Model file for the job. Use its own axes, mm. A direction names the side the tool comes from. Round coordinates to 2 decimals unless told otherwise and drop trailing zeros. Loops run counter-clockwise (first coordinate to the right, second up) from the corner with the lowest first, then second, coordinate; pieces in that order, holes last. Notation, with made-up numbers: M 7.5,-7 L 31.5,-7 A9 ccw 31.5,8 Z; hole C -20.75,49 d8. An arc over 180 degrees is marked long. Answer in a Markdown table with one row per item.
from build123d import *
from OCP.BRepFilletAPI import BRepFilletAPI_MakeChamfer

# Parameters (mm, degrees)
SKETCH_1_W             = 23
SKETCH_1_H             = 37.8
EXTRUDE_1_DEPTH        = 16.4
SKETCH_19_W            = 29
SKETCH_19_H            = 16
EXTRUDE_3_DEPTH        = 6
SKETCH_5_W             = 4
SKETCH_5_H             = 5
EXTRUDE_2_DEPTH        = 13.2
SKETCH_20_W            = 2.9
SKETCH_20_H            = 1.2
SKETCH_20_W_2          = 5.1
EXTRUDE_4_DEPTH        = 5
HOLE_WIZARD_M2_5_1_D   = 2.05
HOLE_WIZARD_M3_6_D     = 2.5
HOLE_WIZARD_M3_6_DEPTH = 7.5
HOLE_WIZARD_M3_6_TIP   = 0.751075774
HOLE_WIZARD_M3_7_D     = 2.5
HOLE_WIZARD_M3_7_DEPTH = 7.5
HOLE_WIZARD_M3_7_TIP   = 0.751075774
HOLE_WIZARD_M3_5_D     = 2.5
SKETCH_15_R            = 5.5
CUT_EXTRUDE_4_DEPTH    = 1.5
HOLE_WIZARD_M3_4_D     = 2.5
HOLE_WIZARD_M3_4_DEPTH = 7.5
HOLE_WIZARD_M3_4_TIP   = 0.751075774
CUT_EXTRUDE_5_REACH    = 66.761
CHAMFER_1_SIZE         = 0.5
CHAMFER_1_SIZE2        = 0.288675135
CHAMFER_2_SIZE         = 0.5
CHAMFER_2_SIZE2        = 0.288675135
SKETCH_25_W            = 10
SKETCH_25_H            = 0.4
CUT_EXTRUDE_6_DEPTH    = 37.8
CHAMFER_3_SIZE         = 0.5


with BuildPart() as part:
    # 草图1 → 拉伸1 (new body)
    with BuildSketch(Plane.XY):
        with Locations((11.5, 18.9)):
            Rectangle(SKETCH_1_W, SKETCH_1_H)
    extrude(amount=EXTRUDE_1_DEPTH)

    # 草图19 → 拉伸3 (add)
    with BuildSketch(Plane.XZ):
        with Locations((11.5, 8.2)):
            Rectangle(SKETCH_19_W, SKETCH_19_H)
    extrude(amount=EXTRUDE_3_DEPTH)

    # 草图5 → 拉伸2 (add)
    with BuildSketch(Plane.XZ.offset(6)):
        with Locations((3.9, 8.2)):
            Rectangle(SKETCH_5_W, SKETCH_5_H)
        with Locations((19.1, 8.2)):
            Rectangle(SKETCH_5_W, SKETCH_5_H)
    extrude(amount=EXTRUDE_2_DEPTH)

    # 草图20 → 拉伸4 (add)
    with BuildSketch(Plane.XY.offset(10.7)):
        with Locations((0.45, -6.6)):
            Rectangle(SKETCH_20_W, SKETCH_20_H)
        with Locations((8.45, -6.6)):
            Rectangle(SKETCH_20_W_2, SKETCH_20_H)
        with Locations((14.55, -6.6)):
            Rectangle(SKETCH_20_W_2, SKETCH_20_H)
        with Locations((22.55, -6.6)):
            Rectangle(SKETCH_20_W, SKETCH_20_H)
    extrude(amount=-EXTRUDE_4_DEPTH)

    # M2.5 螺纹孔1 (through all)
    with Locations(Plane(origin=(21.1, 0, 0), x_dir=(0, 0, -1), z_dir=(1, 0, 0))):
        with Locations((-8.2, -16.2), (-8.2, -10.5)):
            Hole(HOLE_WIZARD_M2_5_1_D / 2)

    # M3 螺纹孔6
    with Locations(Plane(origin=(23, 0, 0), x_dir=(0, 0, -1), z_dir=(1, 0, 0))):
        with Locations((-2.7, 28.8), (-13.7, 18.8)):
            Hole(HOLE_WIZARD_M3_6_D / 2, depth=HOLE_WIZARD_M3_6_DEPTH)
            with Locations((0, 0, -(HOLE_WIZARD_M3_6_DEPTH + HOLE_WIZARD_M3_6_TIP / 2))):  # 118° drill point
                Cone(0, HOLE_WIZARD_M3_6_D / 2, HOLE_WIZARD_M3_6_TIP, mode=Mode.SUBTRACT)

    # M3 螺纹孔7
    with Locations(Plane.ZY):
        with Locations((2.5, 10.8), (13.9, 10.8)):
            Hole(HOLE_WIZARD_M3_7_D / 2, depth=HOLE_WIZARD_M3_7_DEPTH)
            with Locations((0, 0, -(HOLE_WIZARD_M3_7_DEPTH + HOLE_WIZARD_M3_7_TIP / 2))):  # 118° drill point
                Cone(0, HOLE_WIZARD_M3_7_D / 2, HOLE_WIZARD_M3_7_TIP, mode=Mode.SUBTRACT)

    # M3 螺纹孔5 (through all)
    with Locations(Plane.XY.offset(16.4)):
        with Locations((3.5, 14.8), (19.5, 14.8)):
            Hole(HOLE_WIZARD_M3_5_D / 2)

    # 草图15 → 切除-拉伸4 (cut)
    with BuildSketch(Plane(origin=(0, 37.8, 0), x_dir=(1, 0, 0), z_dir=(0, 1, 0))):
        with Locations(Location((11.5, -8.2, 0), (0, 0, 270))):
            Circle(SKETCH_15_R)
    extrude(amount=-CUT_EXTRUDE_4_DEPTH, mode=Mode.SUBTRACT)

    # M3 螺纹孔4
    with Locations(Plane(origin=(0, 37.8, 0), x_dir=(-1, 0, 0), z_dir=(0, 1, 0))):
        with Locations((-2.5, 1.7), (-21.5, 14.2)):
            Hole(HOLE_WIZARD_M3_4_D / 2, depth=HOLE_WIZARD_M3_4_DEPTH)
            with Locations((0, 0, -(HOLE_WIZARD_M3_4_DEPTH + HOLE_WIZARD_M3_4_TIP / 2))):  # 118° drill point
                Cone(0, HOLE_WIZARD_M3_4_D / 2, HOLE_WIZARD_M3_4_TIP, mode=Mode.SUBTRACT)

    # 切除-拉伸5: up to this face of the body (flat: up to its plane)
    cut_extrude_5_end = Plane(part.part.faces().sort_by_distance((-1.5, 0, 8.2))[0])
    # 草图18 → 切除-拉伸5 (cut, up to the picked face)
    with BuildSketch(Plane(origin=(0, 37.8, 0), x_dir=(1, 0, 0), z_dir=(0, 1, 0)), mode=Mode.PRIVATE) as cut_extrude_5_sk1:
        Polygon((23, -10.7), (23, -5.7), (21.5, -5.7), (21.5, -5.1), (17.6, -5.1), (17.6, -11.3), (21.5, -11.3), (21.5, -10.7), align=None)
    cut_extrude_5_tool1 = split(extrude(cut_extrude_5_sk1.sketch, amount=-CUT_EXTRUDE_5_REACH, mode=Mode.PRIVATE), bisect_by=cut_extrude_5_end, keep=Keep.BOTH, mode=Mode.PRIVATE)
    # 草图18 → 切除-拉伸5 (cut, up to the picked face)
    with BuildSketch(Plane(origin=(0, 37.8, 0), x_dir=(1, 0, 0), z_dir=(0, 1, 0)), mode=Mode.PRIVATE) as cut_extrude_5_sk2:
        Polygon((0, -10.7), (1.5, -10.7), (1.5, -11.3), (5.4, -11.3), (5.4, -5.1), (1.5, -5.1), (1.5, -5.7), (0, -5.7), align=None)
    cut_extrude_5_tool2 = split(extrude(cut_extrude_5_sk2.sketch, amount=-CUT_EXTRUDE_5_REACH, mode=Mode.PRIVATE), bisect_by=cut_extrude_5_end, keep=Keep.BOTH, mode=Mode.PRIVATE)
    add(cut_extrude_5_tool1.solids().sort_by(Axis((20.189205, 37.8, 8.2), (0, -1, 0)))[0], mode=Mode.SUBTRACT)
    add(cut_extrude_5_tool2.solids().sort_by(Axis((2.810795, 37.8, 8.2), (0, -1, 0)))[0], mode=Mode.SUBTRACT)

    # 倒角1: one chamfer whose edges measure the first distance from different faces: ONE call of the kernel's chamfer builder (chamfer() names one face for all edges)
    chamfer_1_edges_1 = [part.edges().sort_by_distance(p)[0] for p in [
        (21.5, 18.9, 10.7),
    ]]
    chamfer_1_side_1 = [part.faces().sort_by_distance(p)[0] for p in [
        (21.5, 18.9, 11),
    ]]
    chamfer_1_edges_2 = [part.edges().sort_by_distance(p)[0] for p in [
        (1.5, 18.9, 5.7),
    ]]
    chamfer_1_side_2 = [part.faces().sort_by_distance(p)[0] for p in [
        (1.5, 18.9, 5.4),
    ]]
    chamfer_1 = BRepFilletAPI_MakeChamfer(part.part.solid().wrapped)
    for e in chamfer_1_edges_1:
        chamfer_1.Add(CHAMFER_1_SIZE, CHAMFER_1_SIZE2, e.wrapped, chamfer_1_side_1[0].wrapped)  # the first distance lies on this face
    for e in chamfer_1_edges_2:
        chamfer_1.Add(CHAMFER_1_SIZE, CHAMFER_1_SIZE2, e.wrapped, chamfer_1_side_2[0].wrapped)  # the first distance lies on this face
    add(Compound.cast(chamfer_1.Shape()), mode=Mode.REPLACE)

    # 倒角2: one chamfer whose edges measure the first distance from different faces: ONE call of the kernel's chamfer builder (chamfer() names one face for all edges)
    chamfer_2_edges_1 = [part.edges().sort_by_distance(p)[0] for p in [
        (21.5, 18.9, 5.7),
    ]]
    chamfer_2_side_1 = [part.faces().sort_by_distance(p)[0] for p in [
        (21.5, 18.9, 5.4),
    ]]
    chamfer_2_edges_2 = [part.edges().sort_by_distance(p)[0] for p in [
        (1.5, 18.9, 10.7),
    ]]
    chamfer_2_side_2 = [part.faces().sort_by_distance(p)[0] for p in [
        (1.5, 18.9, 11),
    ]]
    chamfer_2 = BRepFilletAPI_MakeChamfer(part.part.solid().wrapped)
    for e in chamfer_2_edges_1:
        chamfer_2.Add(CHAMFER_2_SIZE, CHAMFER_2_SIZE2, e.wrapped, chamfer_2_side_1[0].wrapped)  # the first distance lies on this face
    for e in chamfer_2_edges_2:
        chamfer_2.Add(CHAMFER_2_SIZE, CHAMFER_2_SIZE2, e.wrapped, chamfer_2_side_2[0].wrapped)  # the first distance lies on this face
    add(Compound.cast(chamfer_2.Shape()), mode=Mode.REPLACE)

    # 草图25 → 切除-拉伸6 (cut)
    with BuildSketch(Plane(origin=(0, 37.8, 0), x_dir=(1, 0, 0), z_dir=(0, 1, 0))):
        with Locations((11.5, -0.2)):
            Rectangle(SKETCH_25_W, SKETCH_25_H)
        with Locations((11.5, -16.2)):
            Rectangle(SKETCH_25_W, SKETCH_25_H)
    extrude(amount=-CUT_EXTRUDE_6_DEPTH, mode=Mode.SUBTRACT)

    # 倒角3
    # the kernel refuses this chamfer: 0.5 mm, written as the material it takes off along each edge
    with BuildSketch(Plane(origin=(23, 0, 16.4), x_dir=(-0.9996219169112968, 0, 0.027495876610589005), z_dir=(0, 1, 0)), Plane(origin=(23, 0, 0), x_dir=(0.02749587661058908, 0, 0.9996219169112968), z_dir=(0, 1, 0))) as chamfer_3_piece_1:
        Polygon((CHAMFER_3_SIZE * 0.999621916911, -CHAMFER_3_SIZE * 0.0274958766106), (-CHAMFER_3_SIZE * 0.0274958766106, -CHAMFER_3_SIZE * 0.999621916911), (0, 0), align=None)
    extrude(amount=39.085841494, mode=Mode.SUBTRACT)
    with BuildSketch(Plane(origin=(0, 39.085841494, 16.4), x_dir=(-0.02749587661058639, 0, -0.9996219169112968), z_dir=(0, -1, 0)), Plane(origin=(0, 39.085841494, 0), x_dir=(0.9996219169112968, 0, -0.027495876610586372), z_dir=(0, -1, 0))) as chamfer_3_piece_2:
        Polygon((CHAMFER_3_SIZE * 0.999621916911, CHAMFER_3_SIZE * 0.0274958766106), (-CHAMFER_3_SIZE * 0.0274958766106, CHAMFER_3_SIZE * 0.999621916911), (0, 0), align=None)
    extrude(amount=39.085841494, mode=Mode.SUBTRACT)


solid = part.part
1. Wall check: probe 1 along Z at (x, y) = (2.5, 34); probe 2 along Y at (x, z) = (3.5, 2.5); probe 3 along Z at (x, y) = (19.5, 18.8). Give the ranges that are in metal, low to high.
Verdict:
| item | result |
|---|---|
| probe 1 | z = 0 to 0.45, 2.95 to 5.1, 11.3 to 16.4 |
| probe 2 | y = -6 to 9.55, 12.05 to 13.55, 16.05 to 37.8 |
| probe 3 | z = 0 to 5.1, 11.3 to 12.45, 14.95 to 16.4 |
2. Saw through at B-B (y = -16.2). Write the cut outline in (x, z) (3 decimals), and give its area (3 significant figures).
Verdict:
| item | result |
|---|---|
| outline | M 1.9,5.7 L 5.9,5.7 L 5.9,7.175 L 1.9,7.175 Z; M 1.9,9.225 L 5.9,9.225 L 5.9,10.7 L 1.9,10.7 Z; M 17.1,5.7 L 21.1,5.7 L 21.1,7.175 L 17.1,7.175 Z; M 17.1,9.225 L 21.1,9.225 L 21.1,10.7 L 17.1,10.7 Z |
| area | 23.6 mm² |
3. Saw through at C-C (z = 8.2). State how many separate pieces and enclosed holes the cut face has, and give its area (3 significant figures).
Verdict:
| item | result |
|---|---|
| separate pieces | 5 |
| enclosed holes | 0 |
| area | 711 mm² |
4. Saw through at A-A (x = 19.5). Write the cut outline in (y, z) (3 decimals).
Verdict:
| item | result |
|---|---|
| outline | M -19.2,5.7 L -6,5.7 L -6,0.2 L 0,0.2 L 0,0 L 13.55,0 L 13.55,5.1 L 0,5.1 L 0,11.3 L 13.55,11.3 L 13.55,16.4 L 0,16.4 L 0,16.2 L -6,16.2 L -6,10.7 L -19.2,10.7 Z; M 16.05,0 L 37.8,0 L 37.8,5.1 L 16.05,5.1 Z; M 16.05,11.3 L 37.8,11.3 L 37.8,16.4 L 16.05,16.4 Z; hole C -16.2,8.2 d2.05; hole C -10.5,8.2 d2.05; hole C 18.8,13.7 d2.5; hole C 28.8,2.7 d2.5 |
5. Tool access for faces 5 (the flat face through (11, 19, 16)), 6 (the flat face through (0, 19, 13)), 7 (the flat face through (15, -7.2, 8)): list every direction of +Z, -Z, +X, -X, +Y, -Y with a clear straight run to the whole face (end or side of a thin tool).
Verdict:
| item | result |
|---|---|
| face 5 | +Z, +Y |
| face 6 | +Z, -Z, -X, +Y |
| face 7 | +Z, -Z, -Y |
6. Pin check, flat tips, straight feed: pin 1 (1.5 mm diameter, centred on y = 7, z = 2.5, fed in from +X); pin 2 (9 mm diameter, centred on x = 21, z = 6.5, fed in from +Y); pin 3 (3 mm diameter, centred on y = 10.8, z = 2.5, fed in from -X); pin 4 (2.5 mm diameter, centred on y = -16.2, z = 8.2, fed in from -X). Stop position of each tip, or through.
Verdict:
| item | result |
|---|---|
| pin 1 | stops at x = 23 |
| pin 2 | stops at y = 37.8 |
| pin 3 | stops at x = 0 |
| pin 4 | stops at x = 1.9 |
7. Mould opens along Y. For faces 1 (the cylindrical face through (3.872, -10.192, 9.178)), 2 (the cylindrical face through (3.872, -15.336, 8.751)), 3 (the flat face through (6, 37.8, 6)), 4 (the flat face through (8, -7.2, 8)) say: +Y half, -Y half, draft (parallel to the pull), parting line (faces both ways), or undercut.
Verdict:
| item | result |
|---|---|
| face 1 | undercut |
| face 2 | undercut |
| face 3 | +Y half |
| face 4 | -Y half |
